Source: CAD feature listing. Evaluate the final solid. Frame: model axes, mm. A direction names the side the tool comes from. Round coordinates to 2 decimals unless told otherwise and drop trailing zeros. Loops run counter-clockwise (first coordinate to the right, second up) from the corner with the lowest first, then second, coordinate; pieces in that order, holes last.
(1) Section B-B, the plane x = -14. Return the cut outline in (y, z).
(2) Section D-D, the plane z = 3. Return the cut outline in (x, y), plus the area to 3 significant figures.
(3) First-contact query: pin 1 Ø6.5 at (x, z) = (11, 16) entering from -Y; pin 2 Ø3 at (x, y) = (13, 9.5) entering from +Z; pin 3 Ø7.5 at (x, z) = (-12, -8.5) entering from +Y; pin 4 Ø6 at (x, z) = (-11.5, 13.5) entering from +Y. Flat tips, straight axial feed; report the tip coordinate or a pass-through.
(4) Mould query, pull axis X, two halves, no side actions, for faces 4 (the cylindrical face through (8.5, 2.5, -5.9)), 5 (the cylindrical face through (-11.52, 12.85, 7.29)), 6 (the flat face through (0, 1, 21.5)), 7 (the cylindrical face through (-16.215, 4.699, 16.176)). Classes: pulls with the +X half, pulls with the -X half, needs draft (parallel to the pull), parting line crosses it, or undercut.
(5) Section A-A, the plane z = -6. Return the cut outline in (x, y), plus the area to 3 significant figures.
(6) Section C-C, the plane z = -2. Return the cut outline in (x, y).
(7) Set-up query: faces 1 (the flat face through (0, 7, 5.5)), 2 (the cylindrical face through (-16.215, 4.699, -6.324)), 3 (the flat face through (14, 5, -6)). Return all of +Z, -Z, +X, -X, +Y, -Y with unobstructed straight access to the full face (end or side cutting, diameter ignored); none if empty.
(8) Material intervals for probe 1 along Z at (x, y) = (11, 1.65); probe 2 along Z at (x, y) = (-9, 3.5); probe 3 along Y at (x, z) = (6, 2), sorted ascending.
```python
from build123d import *

# Parameters (mm, degrees)
BOSS_EXTRUDE1_DEPTH = 10
SKETCH6_W           = 33
SKETCH6_H           = 33
SKETCH6_R           = 2.5
BOSS_EXTRUDE2_DEPTH = 5
SKETCH4_R           = 11.25
CUT_EXTRUDE1_DEPTH  = 16
CUT_EXTRUDE2_REACH  = 29.083
SKETCH5_R           = 1.5
CUT_EXTRUDE3_REACH  = 32.112
SKETCH7_R           = 11.399645817
FILLET1_R           = 1


with BuildPart() as part:
    # Sketch3 → Boss-Extrude1 (new body)
    with BuildSketch(Plane.XY):
        with BuildLine():
            Line((-16.5, 0), (16.5, 0))
            Line((16.5, 0), (16.5, 13.123))
            Line((16.5, 13.123), (11.5, 13.123))
            Line((11.5, 13.123), (5.5, 13.123))
            ThreePointArc((5.5, 13.123), (0, 7.623), (-5.5, 13.123))
            Line((-5.5, 13.123), (-11.5, 13.123))
            Line((-11.5, 13.123), (-16.5, 13.123))
            Line((-16.5, 13.123), (-16.5, 0))
        make_face()
    extrude(amount=BOSS_EXTRUDE1_DEPTH)

    # Sketch6 → Boss-Extrude2 (add)
    with BuildSketch(Plane(origin=(0, 0, 0), x_dir=(-1, 0, 0), z_dir=(0, -1, 0))):
        with Locations((0, -5)):
            Rectangle(SKETCH6_W, SKETCH6_H)
        with Locations(Location((11, -16, 0), (0, 0, 180))):
            Circle(SKETCH6_R, mode=Mode.SUBTRACT)
        with Locations(Location((-11, -16, 0), (0, 0, 180))):
            Circle(SKETCH6_R, mode=Mode.SUBTRACT)
        with Locations(Location((-11, 6, 0), (0, 0, 180))):
            Circle(SKETCH6_R, mode=Mode.SUBTRACT)
        with Locations(Location((11, 6, 0), (0, 0, 180))):
            Circle(SKETCH6_R, mode=Mode.SUBTRACT)
    extrude(amount=-BOSS_EXTRUDE2_DEPTH)

    # Sketch4 → Cut-Extrude1 (cut)
    with BuildSketch(Plane.XY.offset(21.5)):
        with Locations((0, 13.123)):
            Circle(SKETCH4_R)
    extrude(amount=-CUT_EXTRUDE1_DEPTH, mode=Mode.SUBTRACT)

    # Sketch5 → Cut-Extrude2 (cut, up to next)
    with BuildSketch(Plane.XY.offset(5.5), mode=Mode.PRIVATE) as cut_extrude2_sk1:
        with Locations((-5.656854249, 7.466145751)):
            Circle(SKETCH5_R)
    cut_extrude2_tool1 = extrude(cut_extrude2_sk1.sketch, amount=-CUT_EXTRUDE2_REACH, mode=Mode.PRIVATE) & part.part
    # Sketch5 → Cut-Extrude2 (cut, up to next)
    with BuildSketch(Plane.XY.offset(5.5), mode=Mode.PRIVATE) as cut_extrude2_sk2:
        with Locations((5.656854249, 7.466145751)):
            Circle(SKETCH5_R)
    cut_extrude2_tool2 = extrude(cut_extrude2_sk2.sketch, amount=-CUT_EXTRUDE2_REACH, mode=Mode.PRIVATE) & part.part
    add(cut_extrude2_tool1.solids().sort_by_distance((-5.656854, 7.466146, 5.5))[0], mode=Mode.SUBTRACT)
    add(cut_extrude2_tool2.solids().sort_by_distance((5.656854, 7.466146, 5.5))[0], mode=Mode.SUBTRACT)

    # Sketch7 → Cut-Extrude3 (cut, up to next)
    with BuildSketch(Plane(origin=(0, 0, 0), x_dir=(-1, 0, 0), z_dir=(0, 0, -1)), mode=Mode.PRIVATE) as cut_extrude3_sk1:
        with Locations((0, 12.372645817)):
            Circle(SKETCH7_R)
    cut_extrude3_tool1 = extrude(cut_extrude3_sk1.sketch, amount=CUT_EXTRUDE3_REACH, mode=Mode.PRIVATE) & part.part
    add(cut_extrude3_tool1.solids().sort_by_distance((0, 12.372646, 0))[0], mode=Mode.SUBTRACT)

    # Fillet1
    fillet1_edges = [part.edges().sort_by_distance(p)[0] for p in [
        (16.5, 13.123, 5),
        (-16.5, 13.123, 5),
        (16.5, 9.0615, 0),
        (-16.5, 9.0615, 0),
        (-12.597298541, 5, 0),
        (-16.5, 9.0615, 10),
        (16.5, 9.0615, 10),
        (-16.5, 5, -5.75),
        (-16.5, 2.5, -11.5),
        (16.5, 5, -5.75),
        (-12.141637541, 5, 10),
        (13.875, 13.123, 10),
        (-16.5, 5, 15.75),
        (-16.5, 2.5, 21.5),
        (16.5, 5, 15.75),
        (16.5, 2.5, 21.5),
        (16.5, 2.5, -11.5),
        (12.141637541, 5, 10),
        (5.5, 13.123, 2.75),
        (8.375, 13.123, 5.5),
        (-5.5, 13.123, 2.75),
        (11.25, 13.123, 7.75),
        (-11.25, 13.123, 7.75),
        (-8.375, 13.123, 5.5),
        (11, 13.123, 0),
        (12.597298541, 5, 0),
        (-13.875, 13.123, 10),
        (-11, 13.123, 0),
    ]]
    fillet(fillet1_edges, radius=FILLET1_R)


solid = part.part
```
Output values:
1. outline: (0, -11.5) - (5, -11.5) - (5, -1) arc R1 cw to (6, 0) - (12.12, 0) arc R1 ccw to (13.12, 1) - (13.12, 9) arc R1 ccw to (12.12, 10) - (6, 10) arc R1 cw to (5, 11) - (5, 21.5) - (0, 21.5) - close
2. outline: (-16.5, 0) - (16.5, 0) - (16.5, 12.12) arc R1 ccw to (15.5, 13.12) - (6.42, 13.12) arc R1 ccw to (5.43, 12.28) arc R5.5 cw to (-5.43, 12.28) arc R1 ccw to (-6.42, 13.12) - (-15.5, 13.12) arc R1 ccw to (-16.5, 12.12) - close; hole circle Ø3 at (-5.66, 7.47); hole circle Ø3 at (5.66, 7.47)
2. area: 371 mm2
3. pin 1: stops at y = 0
3. pin 2: stops at z = 10
3. pin 3: stops at y = 5
3. pin 4: stops at y = 5.13
4. face 4: undercut
4. face 5: undercut
4. face 6: needs draft
4. face 7: pulls with the -X half
5. outline: (-16.5, 0) - (-13.5, 0) - (-13.5, 5) - (-15.5, 5) arc R1 ccw to (-16.5, 4) - close; (-8.5, 0) - (8.5, 0) - (8.5, 4.78) arc R11.4 cw to (-8.5, 4.78) - close; (13.5, 0) - (16.5, 0) - (16.5, 4) arc R1 ccw to (15.5, 5) - (13.5, 5) - close
5. area: 66.0 mm2
6. outline: (-16.5, 0) - (16.5, 0) - (16.5, 4) arc R1 ccw to (15.5, 5) - (8.69, 5) arc R11.4 cw to (-8.69, 5) - (-15.5, 5) arc R1 ccw to (-16.5, 4) - close
7. face 1: +Z, +Y
7. face 2: -Z, -X, +Y
7. face 3: -Z, +X, -X, +Y
8. probe 1: z = -11.5 to -8.5, -3.5 to 13.5, 18.5 to 21.5
8. probe 2: z = -11.5 to -7.5, -4.5 to 14.5, 17.5 to 21.5
8. probe 3: y = 0 to 6.01, 8.93 to 13.03
